Part print with two shaded views. Sizes in mm from the minimum x, y, z corner. A direction names the side the tool comes from. Coordinates: 2 decimals unless noted, no trailing zeros. Loops run counter-clockwise (first coordinate to the right, second up) from the corner with the lowest first, then second, coordinate; pieces in that order, holes last. Notation, with made-up numbers: (3.5, -3.5) -> (23.5, -3.5) arc R25 ccw to (23.5, 27.5) -> close; hole circle Ø4 at (44.25, 7.5). An arc over 180 degrees is marked (long way). Return JSON: item names as keys, results as strings. Group by question number.
(1) Probe L1, parallel to Y at x = 7, z = 4; L2, parallel to Z at x = 9.75, y = 10; L3, parallel to Y at x = 7, z = 8.25. List the from-to ranges inside material, lowest first.
(2) Saw through at D-D on y = 6.75. Write the cut outline in (x, z) (1 decimal).
(3) Mould opens along Y. For the marked faces 1, 2 and 3 say: pulls with the +Y half, pulls with the -Y half, needs draft (parallel to the pull), parting line crosses it, or undercut.
(4) Saw through at C-C on x = 6.75. Write the cut outline in (y, z) (1 decimal), then the cut area to 3 significant figures.
(5) Tool access for the marked faces 4, 5 and 6: list every direction of +Z, -Z, +X, -X, +Y, -Y with a clear straight run to the whole face (end or side of a thin tool).
(6) Flat gauge pins, fed straight in: pin 1 Ø3 at (y, z) = (9, 1) entering from -X; pin 2 Ø2 at (x, y) = (12.5, 2) entering from -Z; pin 3 Ø3 at (y, z) = (9.5, 1.5) entering from +X (1 decimal); pin 4 Ø5 at (x, z) = (11, 5.5) entering from -Y. Where does each tip first touch, or does it go through?
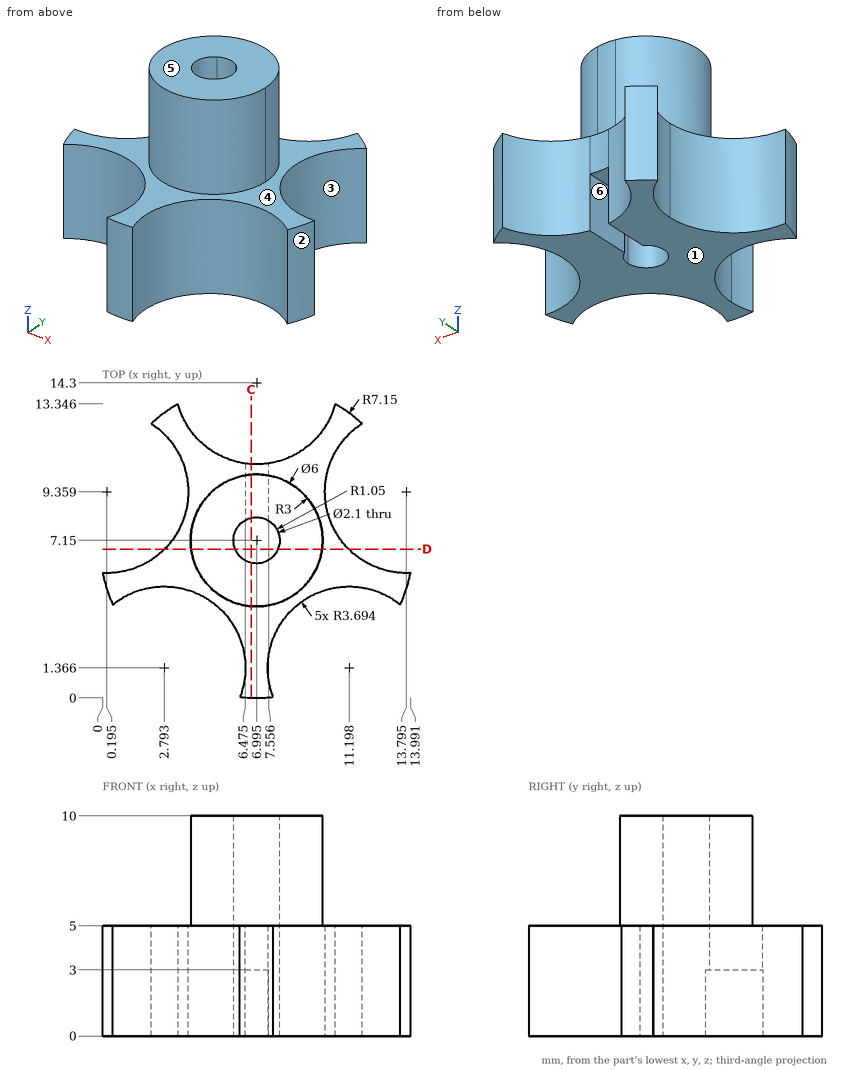
Geometry results:
{
 "1": {"L1": "0 to 6.1, 8.2 to 10.61", "L2": "0 to 5", "L3": "4.15 to 6.1, 8.2 to 10.15"},
 "2": {"outline": "(2.8, 0) -> (6, 0) -> (6, 10) -> (4, 10) -> (4, 5) -> (2.8, 5) -> close; (8, 0) -> (11.2, 0) -> (11.2, 5) -> (10, 5) -> (10, 10) -> (8, 10) -> close"},
 "3": {"face 1": "needs draft", "face 2": "pulls with the -Y half", "face 3": "undercut"},
 "4": {"outline": "(0, 0) -> (6.1, 0) -> (6.1, 10) -> (4.2, 10) -> (4.2, 5) -> (0, 5) -> close; (8.2, 3) -> (10.6, 3) -> (10.6, 5) -> (10.1, 5) -> (10.1, 10) -> (8.2, 10) -> close", "area": "55.2 mm²"},
 "5": {"face 4": "+Z", "face 5": "+Z, +X, -X, +Y, -Y", "face 6": "-Z, +Y"},
 "6": {"pin 1": "x = 3.39", "pin 2": "through", "pin 3": "x = 10.5", "pin 4": "y = 3.94"}
}
